```python
from build123d import *
from build123d.topology import SkipClean

# Parameters (mm, degrees)
ESBO_O1_R                = 1.6
RESSALTO_EXTRUS_O1_DEPTH = 0.75
CORTE_EXTRUS_O1_REACH    = 123.445
ESBO_O2_R                = 9.5
ESBO_O3_R                = 3.5
ESBO_O3_R_2              = 1.6
RESSALTO_EXTRUS_O2_DEPTH = 10


with BuildPart() as part:
    # Esboço1 → Ressalto-extrusão1 (new, symmetric)
    with BuildSketch(Plane(origin=(0, 0, 0), x_dir=(1, 0, 0), z_dir=(0, 1, 0))):
        with BuildLine():
            ThreePointArc((-33.25966317, 13.776603565), (-36, 0), (-33.25966317, -13.776603565))
            ThreePointArc((-33.25966317, -13.776603565), (-33.583097891, -17.060491394), (-36.493241534, -18.615995578))
            ThreePointArc((-36.493241534, -18.615995578), (-72.090991916, -8.566197582), (-109, -11))
            ThreePointArc((-109, -11), (-120, 0), (-109, 11))
            ThreePointArc((-109, 11), (-72.090991916, 8.566197582), (-36.493241534, 18.615995578))
            ThreePointArc((-36.493241534, 18.615995578), (-33.583097891, 17.060491394), (-33.25966317, 13.776603565))
        make_face()
        with Locations(Location((-36.493241534, 15.115995578, 0), (0, 0, 270))):
            Circle(ESBO_O1_R, mode=Mode.SUBTRACT)
        with Locations(Location((-36.493241534, -15.115995578, 0), (0, 0, 270))):
            Circle(ESBO_O1_R, mode=Mode.SUBTRACT)
        with Locations(Location((-95.79, 6, 0), (0, 0, 270))):
            Circle(ESBO_O1_R, mode=Mode.SUBTRACT)
        with Locations(Location((-95.79, -5.96, 0), (0, 0, 270))):
            Circle(ESBO_O1_R, mode=Mode.SUBTRACT)
    extrude(amount=RESSALTO_EXTRUS_O1_DEPTH, both=True)

    # Esboço2 → Corte-extrusão1 (cut, up to next)
    with BuildSketch(Plane(origin=(0, 0.75, 0), x_dir=(1, 0, 0), z_dir=(0, 1, 0)), mode=Mode.PRIVATE) as corte_extrus_o1_sk1:
        with Locations(Location((-109, 0, 0), (0, 0, 270))):
            Circle(ESBO_O2_R)
    corte_extrus_o1_tool1 = extrude(corte_extrus_o1_sk1.sketch, amount=-CORTE_EXTRUS_O1_REACH, mode=Mode.PRIVATE) & part.part
    # Esboço2 → Corte-extrusão1 (cut, up to next)
    with BuildSketch(Plane(origin=(0, 0.75, 0), x_dir=(1, 0, 0), z_dir=(0, 1, 0)), mode=Mode.PRIVATE) as corte_extrus_o1_sk2:
        with BuildLine():
            Line((-88.078445949, 2.757577424), (-52.119636338, 7.831519885))
            ThreePointArc((-52.119636338, 7.831519885), (-44.288116453, 0), (-52.119636338, -7.831519885))
            Line((-52.119636338, -7.831519885), (-88.078445949, -2.757577424))
            ThreePointArc((-88.078445949, -2.757577424), (-90.836023373, 0), (-88.078445949, 2.757577424))
        make_face()
    corte_extrus_o1_tool2 = extrude(corte_extrus_o1_sk2.sketch, amount=-CORTE_EXTRUS_O1_REACH, mode=Mode.PRIVATE) & part.part
    add(corte_extrus_o1_tool1.solids().sort_by_distance((-109, 0.75, 0))[0], mode=Mode.SUBTRACT)
    add(corte_extrus_o1_tool2.solids().sort_by_distance((-64.134293, 0.75, 0))[0], mode=Mode.SUBTRACT)

    # Esboço3 → Ressalto-extrusão2 (add)
    # profile 1 of 4: a face of its own
    with SkipClean():  # the faces are left unmerged after this step: merging them gives an invalid solid
        with BuildSketch(Plane(origin=(0, 0.75, 0), x_dir=(1, 0, 0), z_dir=(0, 1, 0))):
            with Locations(Location((-36.493241534, 15.115995578, 0), (0, 0, 90))):
                Circle(ESBO_O3_R)
            with Locations(Location((-36.493241534, 15.115995578, 0), (0, 0, 270))):
                Circle(ESBO_O3_R_2, mode=Mode.SUBTRACT)
        # profile 2 of 4: a face of its own
        with BuildSketch(Plane(origin=(0, 0.75, 0), x_dir=(1, 0, 0), z_dir=(0, 1, 0))):
            with Locations(Location((-36.493241534, -15.115995578, 0), (0, 0, 270))):
                Circle(ESBO_O3_R)
            with Locations(Location((-36.493241534, -15.115995578, 0), (0, 0, 270))):
                Circle(ESBO_O3_R_2, mode=Mode.SUBTRACT)
        # profile 3 of 4: a face of its own
        with BuildSketch(Plane(origin=(0, 0.75, 0), x_dir=(1, 0, 0), z_dir=(0, 1, 0))):
            with Locations(Location((-95.79, -5.96, 0), (0, 0, 315.511564989))):
                Circle(ESBO_O3_R)
            with Locations(Location((-95.79, -5.96, 0), (0, 0, 270))):
                Circle(ESBO_O3_R_2, mode=Mode.SUBTRACT)
        # profile 4 of 4: a face of its own
        with BuildSketch(Plane(origin=(0, 0.75, 0), x_dir=(1, 0, 0), z_dir=(0, 1, 0))):
            with Locations(Location((-95.79, 6, 0), (0, 0, 123.846033528))):
                Circle(ESBO_O3_R)
            with Locations(Location((-95.79, 6, 0), (0, 0, 270))):
                Circle(ESBO_O3_R_2, mode=Mode.SUBTRACT)
        extrude(amount=RESSALTO_EXTRUS_O2_DEPTH)


solid = part.part
```
Geometry check sheet. Reference: the model listing, model coordinates, mm. A direction names the side the tool comes from. Give positions to 0.01 mm unless a question says otherwise; leave off trailing zeros. Order: outer loops, then holes, each group sorted by start corner. A loop starts at its lowest first (then second) coordinate and runs counter-clockwise, first axis right, second up. Notation, with made-up numbers: (23.25, -29.75) - (42.25, -29.75) arc R19 ccw to (42.25, -21.75) - close; hole circle Ø1 at (80.25, 4.5). An arc over 180 degrees is marked (long way). Answer in a Markdown table with one row per item. Add a question column.
Q1. Tool access check on faces 1 (the flat face through (-64, 0.75, -7)), 2 (the cylindrical face through (-90.835, 0.01, 0.061)), 3 (the flat face through (-95, 10.75, 8)). Record the directions out of +Z, -Z, +X, -X, +Y, -Y that give a thin tool (end or side, any length) a straight path to the whole face; none if there is none.
Q2. Mould release check, pull along Z, two halves, no side actions. Record for faces 4 (the cylindrical face through (-71.574, 0.01, 8.622)), 5 (the cylindrical face through (-99.58, 0.01, -1.24)), 6 (the flat face through (-63, -0.75, 7)), 7 (the cylindrical face through (-99.264, 5.68, 5.533)): pulls with the +Z half, pulls with the -Z half, needs draft (parallel to the pull), parting line crosses it, or undercut.
Q3. Cross-section at C-C, the plane z = -6. Enter the section's corners in (x, y).
Q4. Cross-section at B-B, the plane y = 7.5. Enter the section's corners in (x, z), then the cut area to 3 significant figures.
Q5. Gauge pin test, flat ends, axial feed: pin 1 (4 mm diameter, centred on y = 7, z = 4, fed in from +X); pin 2 (3 mm diameter, centred on y = 8.5, z = -10, fed in from +X); pin 3 (3 mm diameter, centred on x = -76, z = 4.5, fed in from +Y). Record the tip position at first contact, or that the pin passes through.
Q6. Cross-section at D-D, the plane x = -95.79. Enter the section's corners in (y, z), then the cut area to 3 significant figures.
Q7. Material ranges on probe 1 along X at (y, z) = (-0.3, 0); probe 2 along Z at (x, y) = (-95.79, 4.25); probe 3 along X at (y, z) = (2.5, 15), recorded low to high. Write a range as from..to.
Q8. Cross-section at A-A, the plane x = -49. Enter the section's corners in (y, z).
Check values:
| question | item | result |
|---|---|---|
| 1 | face 1 | +Y |
| 1 | face 2 | +Y, -Y |
| 1 | face 3 | +Z, -Z, +X, -X, +Y |
| 2 | face 4 | pulls with the +Z half |
| 2 | face 5 | undercut |
| 2 | face 6 | needs draft |
| 2 | face 7 | undercut |
| 3 | outline | (-118.22, -0.75) - (-116.37, -0.75) - (-116.37, 0.75) - (-118.22, 0.75) - close; (-101.63, -0.75) - (-97.39, -0.75) - (-97.39, 10.75) - (-99.29, 10.75) - (-99.29, 0.75) - (-101.63, 0.75) - close; (-94.19, -0.75) - (-65.1, -0.75) - (-65.1, 0.75) - (-92.29, 0.75) - (-92.29, 10.75) - (-94.19, 10.75) - close; (-47.09, -0.75) - (-35.5, -0.75) - (-35.5, 0.75) - (-47.09, 0.75) - close |
| 4 | outline | circle Ø7 at (-95.79, -6); circle Ø7 at (-95.79, 5.96); circle Ø7 at (-36.49, -15.12); circle Ø7 at (-36.49, 15.12); hole circle Ø3.2 at (-95.79, -6); hole circle Ø3.2 at (-95.79, 5.96); hole circle Ø3.2 at (-36.49, -15.12); hole circle Ø3.2 at (-36.49, 15.12) |
| 4 | area | 122 mm^2 |
| 5 | pin 1 | stops at x = -92.29 |
| 5 | pin 2 | stops at x = -93.34 |
| 5 | pin 3 | stops at y = 0.75 |
| 6 | outline | (-0.75, -8.67) - (0.75, -8.67) - (0.75, -9.5) - (10.75, -9.5) - (10.75, -7.6) - (-0.75, -7.6) - close; (-0.75, -4.4) - (10.75, -4.4) - (10.75, -2.5) - (0.75, -2.5) - (0.75, 2.46) - (10.75, 2.46) - (10.75, 4.36) - (-0.75, 4.36) - close; (-0.75, 7.56) - (10.75, 7.56) - (10.75, 9.46) - (0.75, 9.46) - (0.75, 8.67) - (-0.75, 8.67) - close |
| 6 | area | 92.4 mm^2 |
| 7 | probe 1 | x = -120..-118.5, -99.5..-90.84, -44.29..-36 |
| 7 | probe 2 | z = -9.5..-7.6, -4.4..-2.5, 2.46..4.36, 7.56..9.46 |
| 7 | probe 3 | x = -39.99..-38.09, -34.9..-33 |
| 8 | outline | (-0.75, -13.57) - (0.75, -13.57) - (0.75, -7.18) - (-0.75, -7.18) - close; (-0.75, 7.18) - (0.75, 7.18) - (0.75, 13.57) - (-0.75, 13.57) - close |
